Read the model definition and answer for the solid it produces. Units are mm, in the model's axes. A direction names the side the tool comes from. Round coordinates to 2 decimals unless told otherwise and drop trailing zeros. Loops run counter-clockwise (first coordinate to the right, second up) from the corner with the lowest first, then second, coordinate; pieces in that order, holes last. Notation, with made-up numbers: (61, 63.5) - (102, 63.5) arc R24 cw to (102, 92.5) - close; hole circle Ø7 at (-33, 67.5). An arc over 180 degrees is marked (long way). Use one line per item in the form item = value. Start each with the question number.
```python
from build123d import *

# Parameters (mm, degrees)
F0_W      = 60
F0_H      = 30
F1_DEPTH  = 1.5
F2_W      = 10
F2_H      = 15
F3_DEPTH  = 15
F2_R      = 1.5
F4_DEPTH  = 3
F5_R      = 5
F5_R_2    = 1.5
F6_DEPTH  = 7.5
F7_DEPTH  = 30
F9_DEPTH  = 7.5
F10_W     = 0.3519237886
F10_H     = 30
F10_H_2   = 2.075
F10_H_3   = 27.925
F11_DEPTH = 3
F12_W     = 60.7038475773
F12_H     = 2.5
F13_DEPTH = 3


with BuildPart() as f1:
    # F0 (on Front) → F1 (new body, symmetric)
    with BuildSketch(Plane.XZ):
        Rectangle(F0_W, F0_H)
    extrude(amount=F1_DEPTH, both=True)

    # F2 (on face) → F3 (join)
    with BuildSketch(Plane.XZ.offset(1.5)):
        with Locations((-11, 0)):
            Rectangle(F2_W, F2_H)
        with Locations((11, 0)):
            Rectangle(F2_W, F2_H)
    extrude(amount=F3_DEPTH)

    # F2 (on face) → F4 (cut)
    with BuildSketch(Plane.XZ.offset(1.5)):
        with BuildLine():
            Line((-25.4019237886, 13), (-25.4019237886, 14.5))
            ThreePointArc((-25.4019237886, 14.5), (-26.9019237886, 13), (-25.4019237886, 11.5))
            Line((-25.4019237886, 11.5), (-25.4019237886, 12.925))
            Line((-25.4019237886, 12.925), (-25.4019237886, 13))
        make_face()
        with BuildLine():
            ThreePointArc((-23.9019237886, 13), (-24.3412636169, 14.0606601718), (-25.4019237886, 14.5))
            Line((-25.4019237886, 14.5), (-25.4019237886, 13))
            Line((-25.4019237886, 13), (-25.4019237886, 12.925))
            Line((-25.4019237886, 12.925), (-25.4019237886, 11.5))
            ThreePointArc((-25.4019237886, 11.5), (-24.3412636169, 11.9393398282), (-23.9019237886, 13))
        make_face()
        with BuildLine():
            ThreePointArc((-23.9019237886, -12.925), (-26.4625839604, -11.8643398282), (-25.4019237886, -14.425))
            ThreePointArc((-25.4019237886, -14.425), (-24.3412636169, -13.9856601718), (-23.9019237886, -12.925))
        make_face()
        with Locations((25.4019237886, 12.925)):
            Circle(F2_R)
        with Locations((25.4019237886, -12.925)):
            Circle(F2_R)
        with BuildLine():
            ThreePointArc((-23.9019237886, 0), (-24.3412636169, 1.0606601718), (-25.4019237886, 1.5))
            ThreePointArc((-25.4019237886, 1.5), (-26.4625839604, -1.0606601718), (-23.9019237886, 0))
        make_face()
        with Locations((25.4019237886, 0.075)):
            Circle(F2_R)
    extrude(amount=-F4_DEPTH, mode=Mode.SUBTRACT)

    # F5 (on Right) → F6 (cut, symmetric)
    with BuildSketch(Plane.YZ):
        with Locations((-9, 0)):
            Circle(F5_R)
        with Locations((-9, 0)):
            Circle(F5_R_2, mode=Mode.SUBTRACT)
    extrude(amount=F6_DEPTH, both=True, mode=Mode.SUBTRACT)

    # F7 (cut, symmetric): a face of the model
    f7_faces = [f1.faces().sort_by_distance(p)[0] for p in [
        (-6, -9, 0),
    ]]
    extrude(f7_faces, amount=F7_DEPTH, both=True, mode=Mode.SUBTRACT)

    # F8 (on Right) → F9 (cut, symmetric)
    with BuildSketch(Plane.YZ):
        Polygon((-9, 5), (-16.5, 5), (-16.5, -5), (-9, -5), (-9, 0), align=None)
    extrude(amount=F9_DEPTH, both=True, mode=Mode.SUBTRACT)

    # F10 (on face) → F11 (join)
    with BuildSketch(Plane(origin=(0, 1.5, 0), x_dir=(-1, 0, 0), z_dir=(0, 1, 0))):
        with Locations((30.1759618943, 0)):
            Rectangle(F10_W, F10_H)
        with Locations((-30.1759618943, -13.9625)):
            Rectangle(F10_W, F10_H_2)
        with Locations((-30.1759618943, 1.0375)):
            Rectangle(F10_W, F10_H_3)
    extrude(amount=-F11_DEPTH)

    # F12 (on face) → F13 (join)
    with BuildSketch(Plane(origin=(0, 1.5, 0), x_dir=(-1, 0, 0), z_dir=(0, 1, 0))):
        with Locations((0, 16.25)):
            Rectangle(F12_W, F12_H)
        with Locations((0, -16.25)):
            Rectangle(F12_W, F12_H)
    extrude(amount=-F13_DEPTH)


solid = f1.part
```
1) Determine the mould class of faces 4 (the flat face through (-11, -9, -7.5)), 5 (the flat face through (0, 1.5, 0)), 6 (the flat face through (7, -13, 5)) for opening direction Z: +Z half, -Z half, draft (parallel to the pull), parting line (faces both ways), or undercut.
2) A cutting plane is placed at A-A on y = -3. Write down the section's boundary in (x, z), plus the area to 3 significant figures.
3) For faces 1 (the flat face through (-11, -9, 7.5)), 2 (the flat face through (7.5, -12, 0)), 3 (the flat face through (16, -7, 0)), determine the directions among +Z, -Z, +X, -X, +Y, -Y from which every point of the face is accessible in a straight line to the end or side of a thin tool.
4) A cutting plane is placed at C-C on x = -2. Write down the section's boundary in (y, z).
5) Flat-ended cylindrical pins translate along their axes: pin 1 (2.5 mm diameter, centred on y = -9, z = 0, fed in from -X); pin 2 (4 mm diameter, centred on y = -9, z = 0, fed in from -X); pin 3 (3 mm diameter, centred on x = 9.5, y = -9, fed in from -Z); pin 4 (4.5 mm diameter, centred on y = -10, z = -0.5, fed in from +X). Find the tip coordinate at first contact, or state that the pin passes through.
6) A cutting plane is placed at B-B on z = 6. Write down the section's boundary in (x, y), plus the area to 3 significant figures.
7) Straight lines are drawn through the part: line 1 (X direction, y = -1.25, z = 13); line 2 (X direction, y = -1, z = -14); line 3 (X direction, y = -6.75, z = -7). For each, find the intervals that lie inside material, in ascending order. Write a range as from..to.
Checks:
q1.face_4 = -Z half
q1.face_5 = draft
q1.face_6 = undercut
q2.outline = (-16, -7.5) - (-6, -7.5) - (-6, 7.5) - (-16, 7.5) - close; (6, -7.5) - (16, -7.5) - (16, 7.5) - (6, 7.5) - close
q2.area = 300 mm²
q3.face_1 = +Z, +X, -X, -Y
q3.face_2 = -Y
q3.face_3 = +Z, -Z, +X, -Y
q4.outline = (-1.5, -17.5) - (1.5, -17.5) - (1.5, 17.5) - (-1.5, 17.5) - close
q5.pin_1 = through
q5.pin_2 = -16
q5.pin_3 = -7.5
q5.pin_4 = 16
q6.outline = (-30.35, -1.5) - (-16, -1.5) - (-16, -16.5) - (-6, -16.5) - (-6, -1.5) - (6, -1.5) - (6, -16.5) - (16, -16.5) - (16, -1.5) - (30.35, -1.5) - (30.35, 1.5) - (-30.35, 1.5) - close
q6.area = 482 mm²
q7.line_1 = -30.35..-26.9, -23.9..23.9, 26.9..30.35
q7.line_2 = -30.35..-26.45, -24.36..24.36, 26.45..30.35
q7.line_3 = -16..-6, 6..16
